Answer from the drawing. Dimensions are ordinates in mm from the lowest x, y and z of the part. A direction names the side the tool comes from. Give positions to 0.01 mm unless a question says otherwise; leave off trailing zeros. Order: outer loops, then holes, each group sorted by start corner. A loop starts at its lowest first (then second) coordinate and runs counter-clockwise, first axis right, second up. Notation, with made-up numbers: M 73.5,88 L 93.5,88 A10 ccw 93.5,96 Z; hole C 1,39 d3. An arc over 180 degrees is marked long. One line per item, written item: value.
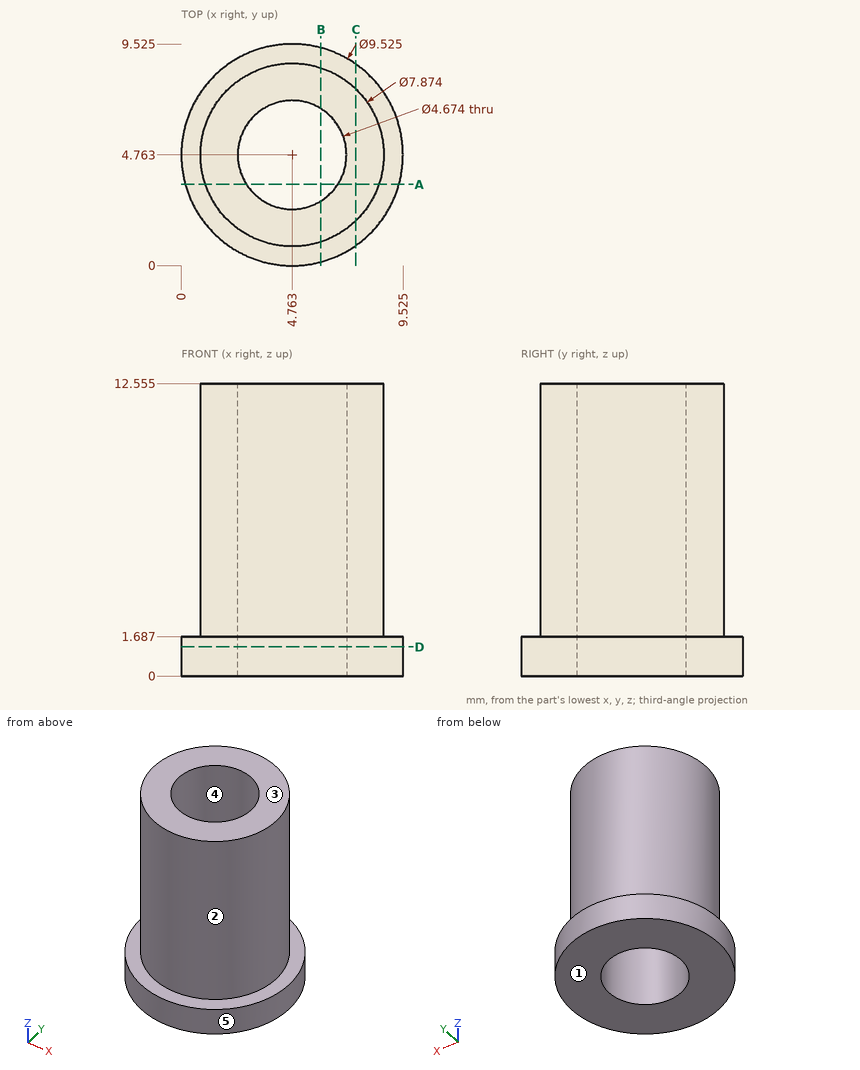
(1) Determine the mould class of the marked faces 3, 4 and 5 for opening direction Y: pulls with the +Y half, pulls with the -Y half, needs draft (parallel to the pull), parting line crosses it, or undercut.
Findings:
face 3: needs draft
face 4: undercut
face 5: parting line crosses it
(2) Which of the six approach directions +Z, -Z, +X, -X, +Y, -Y give full straight-line access (tool end or side, diameter ignored) to the marked faces 1 and 2?
Findings:
face 1: -Z, +X, -X, +Y, -Y
face 2: +Z
(3) Find the intervals of material crossed by probe 1 along Y at (x, z) = (4.75, 6.75) (1 decimal); probe 2 along Z at (x, y) = (2.5, 0.75), in increasing order. Write a range as from..to.
Findings:
probe 1: y = 0.8..2.4, 7.1..8.7
probe 2: z = 0..1.69
(4) Section A-A, the plane y = 3.5 is taken. Give the vertices of the cut face in (x, z) (1 decimal).
Findings:
outline: M 0.2,0 L 2.8,0 L 2.8,12.6 L 1,12.6 L 1,1.7 L 0.2,1.7 Z; M 6.7,0 L 9.4,0 L 9.4,1.7 L 8.5,1.7 L 8.5,12.6 L 6.7,12.6 Z
(5) Given P1, Ø4, axis at y = 7.5, z = 2, coming from the +X side; P2, Ø2, axis at x = 3.5, z = 2.5, coming from the +Y side, each flat-ended and moving along its own axis, determine where each tip first touches the part or whether it passes through.
Findings:
P1: stops at x = 9.46
P2: stops at y = 9.48
(6) Section D-D, the plane z = 1.25 is taken. Give the vertices of the cut face in (x, y) (1 decimal), then the cut area to 3 significant figures.
Findings:
outline: C 4.8,4.8 d9.5; hole C 4.8,4.8 d4.7
area: 54.1 mm^2
(7) Section C-C, the plane x = 7.5 is taken. Give the vertices of the cut face in (y, z) (1 decimal).
Findings:
outline: M 0.9,0 L 8.7,0 L 8.7,1.7 L 7.6,1.7 L 7.6,12.6 L 1.9,12.6 L 1.9,1.7 L 0.9,1.7 Z
